from build123d import *

# Parameters (mm, degrees)
F1_DEPTH = 6.35
F2_DEPTH = 9.525
F0_R     = 23.315742
F3_DEPTH = 0.635
F0_R_2   = 20.775742
F4_DEPTH = 1.27


with BuildPart() as f1:
    # F0 (on Top) → F1 (new body, symmetric)
    with BuildSketch(Plane.XY):
        with BuildLine():
            Line((57.15, 44.45), (-57.15, 44.45))
            ThreePointArc((-57.15, 44.45), (-61.640128, 42.590128), (-63.5, 38.1))
            Line((-63.5, 38.1), (-63.5, -38.1))
            ThreePointArc((-63.5, -38.1), (-61.640128, -42.590128), (-57.15, -44.45))
            Line((-57.15, -44.45), (57.15, -44.45))
            ThreePointArc((57.15, -44.45), (61.640128, -42.590128), (63.5, -38.1))
            Line((63.5, -38.1), (63.5, 38.1))
            ThreePointArc((63.5, 38.1), (61.640128, 42.590128), (57.15, 44.45))
        make_face()
        with BuildLine():
            Line((54.61, -41.91), (-54.61, -41.91))
            ThreePointArc((-54.61, -41.91), (-59.100128, -40.050128), (-60.96, -35.56))
            Line((-60.96, -35.56), (-60.96, 35.56))
            ThreePointArc((-60.96, 35.56), (-59.100128, 40.050128), (-54.61, 41.91))
            Line((-54.61, 41.91), (54.61, 41.91))
            ThreePointArc((54.61, 41.91), (59.100128, 40.050128), (60.96, 35.56))
            Line((60.96, 35.56), (60.96, -35.56))
            ThreePointArc((60.96, -35.56), (59.100128, -40.050128), (54.61, -41.91))
        make_face(mode=Mode.SUBTRACT)
    extrude(amount=F1_DEPTH, both=True)

    # F0 (on Top) → F2 (join, symmetric)
    with BuildSketch(Plane.XY):
        with BuildLine():
            ThreePointArc((-60.96, -35.56), (-59.100128, -40.050128), (-54.61, -41.91))
            Line((-54.61, -41.91), (54.61, -41.91))
            ThreePointArc((54.61, -41.91), (59.100128, -40.050128), (60.96, -35.56))
            Line((60.96, -35.56), (60.96, 35.56))
            ThreePointArc((60.96, 35.56), (59.100128, 40.050128), (54.61, 41.91))
            Line((54.61, 41.91), (-54.61, 41.91))
            ThreePointArc((-54.61, 41.91), (-59.100128, 40.050128), (-60.96, 35.56))
            Line((-60.96, 35.56), (-60.96, -35.56))
        make_face()
        with BuildLine():
            ThreePointArc((-58.42, 33.02), (-56.560128, 37.510128), (-52.07, 39.37))
            Line((-52.07, 39.37), (52.07, 39.37))
            ThreePointArc((52.07, 39.37), (56.560128, 37.510128), (58.42, 33.02))
            Line((58.42, 33.02), (58.42, -33.02))
            ThreePointArc((58.42, -33.02), (56.560128, -37.510128), (52.07, -39.37))
            Line((52.07, -39.37), (-52.07, -39.37))
            ThreePointArc((-52.07, -39.37), (-56.560128, -37.510128), (-58.42, -33.02))
            Line((-58.42, -33.02), (-58.42, 33.02))
        make_face(mode=Mode.SUBTRACT)
    extrude(amount=F2_DEPTH, both=True)

    # F0 (on Top) → F3 (join, symmetric)
    with BuildSketch(Plane.XY):
        with BuildLine():
            Line((52.07, 39.37), (-52.07, 39.37))
            ThreePointArc((-52.07, 39.37), (-56.560128, 37.510128), (-58.42, 33.02))
            Line((-58.42, 33.02), (-58.42, -33.02))
            ThreePointArc((-58.42, -33.02), (-56.560128, -37.510128), (-52.07, -39.37))
            Line((-52.07, -39.37), (52.07, -39.37))
            ThreePointArc((52.07, -39.37), (56.560128, -37.510128), (58.42, -33.02))
            Line((58.42, -33.02), (58.42, 33.02))
            ThreePointArc((58.42, 33.02), (56.560128, 37.510128), (52.07, 39.37))
        make_face()
        Circle(F0_R, mode=Mode.SUBTRACT)
    extrude(amount=F3_DEPTH, both=True)

    # F0 (on Top) → F4 (join)
    with BuildSketch(Plane.XY):
        Circle(F0_R)
        Circle(F0_R_2, mode=Mode.SUBTRACT)
    extrude(amount=-F4_DEPTH)


solid = f1.part
For this review, take the finished solid that the model builds, in its own axes (mm). A direction names the side the tool comes from. Round coordinates to 2 decimals unless told otherwise and drop trailing zeros. Loops run counter-clockwise (first coordinate to the right, second up) from the corner with the lowest first, then second, coordinate; pieces in that order, holes last. Notation, with made-up numbers: (73, -12) - (87, -12) arc R21 cw to (87, 1) - close; hole circle Ø11 at (-14, 7). An arc over 180 degrees is marked (long way). Put each result on its own line as item: value. Start each with the question number.
1. For probe 1 along Y at (x, z) = (0, -0.9); probe 2 along X at (y, z) = (-20.5, -5.25); probe 3 along X at (y, z) = (-19, 8.25), list the stretches that pass through material, from the lowest coordinate up. Write a range as [from, to].
2. Mouldability with a two-part tool opening along Y and no side actions: class faces 1 (the flat face through (63.5, -1, 0)), 2 (the cylindrical face through (-59.05, 40.1, 7.96)), 3 (the flat face through (58.42, 0, -5)), 4 (the flat face through (58.42, 0, 5)) as +Y half, -Y half, draft (parallel to the pull), parting line (faces both ways), or undercut.
3. Consider section D-D on x = -50.5. State the section outline as (y, z) points (3 decimals).
4. Consider section B-B on z = 8. State the section outline as (x, y) points, plus the area to 3 significant figures.
5. Insertion check: P1, Ø1, axis at x = -7.5, z = 7.5, coming from the -Y side; P2, Ø23.5, axis at x = -3, y = 0.5, coming from the +Z side; P3, Ø1, axis at y = -3.5, z = -8.5, coming from the +X side; P4, Ø3.5, axis at y = 17, z = 8.5, coming from the -X side. Each pin has a flat end and moves straight along its axis. Give the tip position at first contact, or say it passes through.
6. For faces 5 (the flat face through (-60.96, 0, -8)), 6 (the flat face through (60.96, 0, 8)), 7 (the flat face through (-58.42, 0, 5)), 8 (the cylindrical face through (56.61, -37.46, -5.02)), list the 3-axis set-ups (+Z, -Z, +X, -X, +Y, -Y) from which the entire face can be reached by the end or side of a thin tool; tool diameter is ignored.
Result sheet:
1. probe 1: [-44.45, -39.37], [-23.32, -20.78], [20.78, 23.32], [39.37, 44.45]
1. probe 2: [-63.5, -58.42], [58.42, 63.5]
1. probe 3: [-60.96, -58.42], [58.42, 60.96]
2. face 1: draft
2. face 2: +Y half
2. face 3: undercut
2. face 4: undercut
3. outline: (-44.45, -6.35) - (-41.91, -6.35) - (-41.91, -9.525) - (-39.37, -9.525) - (-39.37, -0.635) - (39.37, -0.635) - (39.37, -9.525) - (41.91, -9.525) - (41.91, -6.35) - (44.45, -6.35) - (44.45, 6.35) - (41.91, 6.35) - (41.91, 9.525) - (39.37, 9.525) - (39.37, 0.635) - (-39.37, 0.635) - (-39.37, 9.525) - (-41.91, 9.525) - (-41.91, 6.35) - (-44.45, 6.35) - close
4. outline: (-60.96, -35.56) arc R6.35 ccw to (-54.61, -41.91) - (54.61, -41.91) arc R6.35 ccw to (60.96, -35.56) - (60.96, 35.56) arc R6.35 ccw to (54.61, 41.91) - (-54.61, 41.91) arc R6.35 ccw to (-60.96, 35.56) - close; hole (-58.42, -33.02) arc R6.35 ccw to (-52.07, -39.37) - (52.07, -39.37) arc R6.35 ccw to (58.42, -33.02) - (58.42, 33.02) arc R6.35 ccw to (52.07, 39.37) - (-52.07, 39.37) arc R6.35 ccw to (-58.42, 33.02) - close
4. area: 1,020 mm^2
5. P1: y = -41.91
5. P2: through
5. P3: x = 60.96
5. P4: x = -60.96
6. face 5: -Z, -X, +Y, -Y
6. face 6: +Z, +X, +Y, -Y
6. face 7: +Z
6. face 8: -Z
